Design review of the part built by this model. Coordinates are the model's own, in mm. Face numbers are marked on the shaded views. Coordinates: 2 decimals unless noted, no trailing zeros. Order: outer loops, then holes, each group sorted by start corner. A loop starts at its lowest first (then second) coordinate and runs counter-clockwise, first axis right, second up.
from build123d import *


with BuildPart() as part:
    # Esquisse1 → Révolution1 (revolve)
    with BuildSketch(Plane.XY, mode=Mode.PRIVATE) as r_volution1_sk:
        with BuildLine():
            Line((0, 8.75), (0, 12))
            ThreePointArc((0, 12), (-0.146446609, 12.353553391), (-0.5, 12.5))
            Line((-0.5, 12.5), (-2.5, 12.5))
            Line((-2.5, 12.5), (-2.5, 13))
            Line((-2.5, 13), (0.4, 13))
            ThreePointArc((0.4, 13), (0.470710678, 12.970710678), (0.5, 12.9))
            Line((0.5, 12.9), (0.5, 8.35))
            ThreePointArc((0.5, 8.35), (0.324264069, 7.925735931), (-0.1, 7.75))
            Line((-0.1, 7.75), (-2, 7.75))
            Line((-2, 7.75), (-2, 8.25))
            Line((-2, 8.25), (-0.5, 8.25))
            ThreePointArc((-0.5, 8.25), (-0.146446609, 8.396446609), (0, 8.75))
        make_face()
    revolve(r_volution1_sk.sketch.rotate(Axis((-5.956424792, 0, 0), (1, 0, 0)), 90), axis=Axis((-5.956424792, 0, 0), (1, 0, 0)))  # turned: the seam where the file's is


solid = part.part
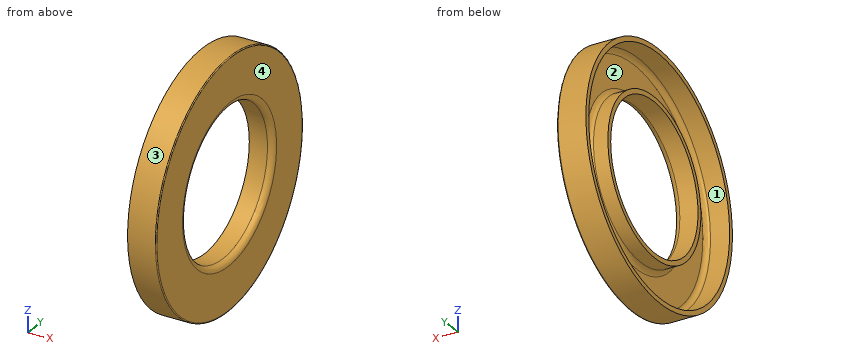
1. Insertion check: pin 1 (1.5 mm diameter, centred on y = -6.5, z = -6, fed in from -X); pin 2 (1.5 mm diameter, centred on y = 5.5, z = -7.5, fed in from -X). Each pin has a flat end and moves straight along its axis. Give the tip position at first contact, or say it passes through.
2. To check wall thickness, follow line 1 (Y direction, x = -1.2, z = 0); line 2 (Y direction, x = -0.9, z = 7); line 3 (Z direction, x = -1, y = 3.75). State the ranges of each line that lie inside material, in increasing order.
3. Add section C-C (x = -1). Give the boundary of the cut face in (y, z), and give its area (3 significant figures).
4. Add section A-A (y = 0). Give the boundary of the cut face in (x, z).
5. Mouldability with a two-part tool opening along Z and no side actions: class the marked faces 1, 2, 3 and 4 as pulls with the +Z half, pulls with the -Z half, needs draft (parallel to the pull), parting line crosses it, or undercut.
Solution:
1. pin 1: stops at x = -2
1. pin 2: stops at x = -0.04
2. line 1: y = -13 to -12.5, -8.25 to -7.75, 7.75 to 8.25, 12.5 to 13
2. line 2: y = -10.95 to -10.36, -4.37 to -3.33, 3.33 to 4.37, 10.36 to 10.95
2. line 3: z = -12.45 to -11.92, -7.35 to -6.78, 6.78 to 7.35, 11.92 to 12.45
3. outline: circle Ø26 at (0, 0); circle Ø16.5 at (0, 0); hole circle Ø25 at (0, 0); hole circle Ø15.5 at (0, 0)
3. area: 65.2 mm2
4. outline: (-2.5, -13) - (0.4, -13) arc R0.1 ccw to (0.5, -12.9) - (0.5, -8.35) arc R0.6 ccw to (-0.1, -7.75) - (-2, -7.75) - (-2, -8.25) - (-0.5, -8.25) arc R0.5 cw to (0, -8.75) - (0, -12) arc R0.5 cw to (-0.5, -12.5) - (-2.5, -12.5) - close; (-2.5, 12.5) - (-0.5, 12.5) arc R0.5 cw to (0, 12) - (0, 8.75) arc R0.5 cw to (-0.5, 8.25) - (-2, 8.25) - (-2, 7.75) - (-0.1, 7.75) arc R0.6 ccw to (0.5, 8.35) - (0.5, 12.9) arc R0.1 ccw to (0.4, 13) - (-2.5, 13) - close
5. face 1: undercut
5. face 2: undercut
5. face 3: parting line crosses it
5. face 4: needs draft
